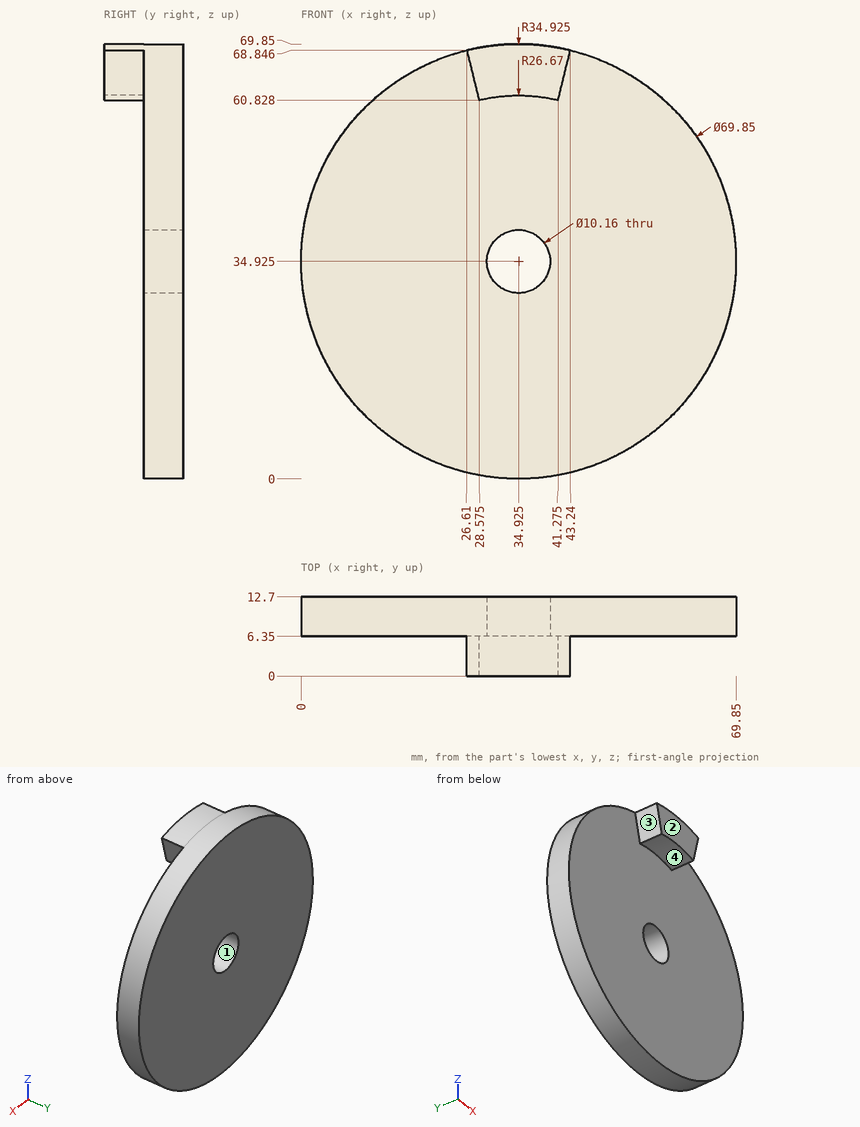
Verification items for this drawing (mm, ordinates from the low corner). Give positions to 0.01 mm unless a question says otherwise; leave off trailing zeros. Write item = value, one per line.
Item 1: Gauge pin test, flat ends, axial feed: pin 1 (6 mm diameter, centred on y = 10.5, z = 14.5, fed in from -X); pin 2 (6 mm diameter, centred on x = 24, y = 11, fed in from +Z). Record the tip position at first contact, or that the pin passes through.
Output:
pin_1 = 4.66
pin_2 = 68.94
Item 2: Release check for a two-part mould opening along X. For the marked faces 1, 2, 3 and 4 record: +X half, -X half, draft (parallel to the pull), parting line (faces both ways), or undercut.
Output:
face_1 = undercut
face_2 = draft
face_3 = -X half
face_4 = undercut
Item 3: Scan lines: probe 1 along Y at (x, z) = (27.5, 52); probe 2 along X at (y, z) = (8.75, 30.5) (1 decimal); probe 3 along Z at (x, y) = (33, 12) (1 decimal). Record each from-to range of solid material in increasing order. Write a range as from..to.
Output:
probe_1 = 6.35..12.7
probe_2 = 0.3..32.4, 37.4..69.6
probe_3 = 0.1..30.2, 39.6..69.8
